```python
from build123d import *

# Parameters (mm, degrees)
F5_W = 0.5
F5_H = 2


with BuildPart() as f3:
    # F3: sweep along a path in F2
    with BuildLine(Plane.XY) as f3_path:
        Line((-8.2, 0), (-7.9205917756, 2.1223161698))
        Line((-7.9205917756, 2.1223161698), (-7.101408311, 4.1))
        Line((-7.101408311, 4.1), (-5.7982756057, 5.7982756057))
        Line((-5.7982756057, 5.7982756057), (-4.1, 7.101408311))
        Line((-4.1, 7.101408311), (-2.1223161698, 7.9205917756))
        Line((-2.1223161698, 7.9205917756), (0, 8.2))
        Line((0, 8.2), (2.1223161698, 7.9205917756))
        Line((2.1223161698, 7.9205917756), (4.1, 7.101408311))
        Line((4.1, 7.101408311), (5.7982756057, 5.7982756057))
        Line((5.7982756057, 5.7982756057), (7.101408311, 4.1))
        Line((7.101408311, 4.1), (7.9205917756, 2.1223161698))
        Line((7.9205917756, 2.1223161698), (8.2, 0))
        Line((8.2, 0), (7.9205917756, -2.1223161698))
        Line((7.9205917756, -2.1223161698), (7.101408311, -4.1))
        Line((7.101408311, -4.1), (5.7982756057, -5.7982756057))
        Line((5.7982756057, -5.7982756057), (4.1, -7.101408311))
        Line((4.1, -7.101408311), (2.1223161698, -7.9205917756))
        Line((2.1223161698, -7.9205917756), (0, -8.2))
        Line((0, -8.2), (-2.1223161698, -7.9205917756))
        Line((-2.1223161698, -7.9205917756), (-4.1, -7.101408311))
        Line((-4.1, -7.101408311), (-5.7982756057, -5.7982756057))
        Line((-5.7982756057, -5.7982756057), (-7.101408311, -4.1))
        Line((-7.101408311, -4.1), (-7.9205917756, -2.1223161698))
        Line((-7.9205917756, -2.1223161698), (-8.2, 0))
    # F1 (on Front) → F3 (sweep)
    with BuildSketch(Plane.XZ):
        Polygon((-8.255, -1), (-8.255, 1), (-8.735039811, 0.6112714258), (-8.8155152209, 0), (-8.735039811, -0.6112714258), align=None)
    sweep(path=f3_path.line, transition=Transition.RIGHT)

    # F6: sweep along a path in F0
    with BuildLine(Plane.XY) as f6_path:
        CenterArc((0, 0), 8.255, 0, 360)
    # F5 (on Front) → F6 (sweep, cut)
    with BuildSketch(Plane.XZ):
        with Locations((-8.005, 0)):
            Rectangle(F5_W, F5_H)
    sweep(path=f6_path.line, mode=Mode.SUBTRACT)

    # F9: sweep along a path in F7
    with BuildLine(Plane.XY) as f9_path:
        Line((-8.255, -2.2119205835), (-8.255, 2.2119205835))
        Line((-8.255, 2.2119205835), (-6.0430794165, 6.0430794165))
        Line((-6.0430794165, 6.0430794165), (-2.2119205835, 8.255))
        Line((-2.2119205835, 8.255), (2.2119205835, 8.255))
        Line((2.2119205835, 8.255), (6.0430794165, 6.0430794165))
        Line((6.0430794165, 6.0430794165), (8.255, 2.2119205835))
        Line((8.255, 2.2119205835), (8.255, -2.2119205835))
        Line((8.255, -2.2119205835), (6.0430794165, -6.0430794165))
        Line((6.0430794165, -6.0430794165), (2.2119205835, -8.255))
        Line((2.2119205835, -8.255), (-2.2119205835, -8.255))
        Line((-2.2119205835, -8.255), (-6.0430794165, -6.0430794165))
        Line((-6.0430794165, -6.0430794165), (-8.255, -2.2119205835))
    # F8 (on Front) → F9 (sweep)
    with BuildSketch(Plane.XZ):
        Polygon((-8.255, -0.75), (-8.255, 0.75), (-8.9203372997, 0), align=None)
    sweep(path=f9_path.line, transition=Transition.RIGHT)


solid = f3.part
```
Geometry: final body of the model. Coordinates: model frame, mm. Round coordinates to 2 decimals unless told otherwise and drop trailing zeros. Order: outer loops, then holes, each group sorted by start corner. A loop starts at its lowest first (then second) coordinate and runs counter-clockwise, first axis right, second up. Notation, with made-up numbers: M 78,15 L 128,15 A28 cw 128,45 Z; hole C 12.5,-2 d9. An arc over 180 degrees is marked long. Use one line per item in the form item = value. Start each with the question number.
Q1. Mould query, pull axis Y, two halves, no side actions, for faces 1 (the face through (3.2, -7.8, -0.8)), 2 (the face through (3.809, -7.324, -0.014)), 3 (the face through (5.17, 6.66, -0.8)). Classes: +Y half, -Y half, draft (parallel to the pull), parting line (faces both ways), or undercut.
Q2. Material intervals for line 1 (X direction, y = -1.25, z = -0.55); line 2 (Y direction, x = 5.5, z = -0.2); line 3 (X direction, y = 0, z = 0.35) (3 decimals), sorted ascending. Write a range as [from, to].
Q3. Pin query (flat end, axial travel): pin 1 Ø10 at (x, y) = (-2, 2.5) entering from +Z. Return the tip coordinate at first contact, or that it passes through.
Q4. Cut plane A-A (y = 5.5). Return loops of the section in (x, z).
Q5. Cut plane B-B (x = 2.75). Return loops of the section in (y, z).
Geometry results:
q1.face_1 = -Y half
q1.face_2 = undercut
q1.face_3 = +Y half
q2.line_1 = [-8.58, -8.16], [8.16, 8.58]
q2.line_2 = [-6.92, -6.16], [6.16, 6.92]
q2.line_3 = [-8.769, -8.255], [8.255, 8.769]
q3.pin_1 = through
q4.outline = M -7.12,0 L -6.73,-0.38 L -6.7,-0.61 L -6.16,-0.96 L -6.16,0.96 L -6.7,0.61 L -6.73,0.38 Z; M 6.16,-0.96 L 6.7,-0.61 L 6.73,-0.38 L 7.12,0 L 6.73,0.38 L 6.7,0.61 L 6.16,0.96 Z
q5.outline = M -8.71,0 L -8.26,-0.44 L -8.23,-0.61 L -7.78,-0.95 L -7.78,0.95 L -8.23,0.61 L -8.26,0.44 Z; M 7.78,-0.95 L 8.23,-0.61 L 8.26,-0.44 L 8.71,0 L 8.26,0.44 L 8.23,0.61 L 7.78,0.95 Z
